Model file for the job. Use its own axes, mm. A direction names the side the tool comes from. Round coordinates to 2 decimals unless told otherwise and drop trailing zeros. Loops run counter-clockwise (first coordinate to the right, second up) from the corner with the lowest first, then second, coordinate; pieces in that order, holes last.
from build123d import *
from OCP.BRepFilletAPI import BRepFilletAPI_MakeChamfer

# Parameters (mm, degrees)
BOSS_EXTRUDE1_DEPTH = 11.1125
FILLET1_R           = 6.35
FILLET2_R           = 5.715
SKETCH2_R           = 2.794
BOSS_EXTRUDE2_DEPTH = 3.175
BOSS_EXTRUDE3_DEPTH = 1.27
SKETCH4_W           = 1.016
SKETCH4_H           = 4.445
CUT_EXTRUDE2_DEPTH  = 20.997176622
CHAMFER1_SIZE       = 0.79375
CHAMFER1_SIZE2      = 0.458271776


# Some blends are built 0.0001 mm under size
with BuildPart() as part:
    # Sketch1 → Boss-Extrude1 (new body)
    with BuildSketch(Plane.XY):
        with BuildLine():
            Line((3.302, 0), (15.367, 0))
            Line((15.367, 0), (15.367, -6.35))
            Line((15.367, -6.35), (-6.477, -6.35))
            Line((-6.477, -6.35), (-6.477, 0))
            Line((-6.477, 0), (-3.302, 0))
            ThreePointArc((-3.302, 0), (0, -3.302), (3.302, 0))
        make_face()
    extrude(amount=BOSS_EXTRUDE1_DEPTH)

    # Fillet1
    fillet1_edges = [part.edges().sort_by_distance(p)[0] for p in [
        (-6.477, -6.35, 5.55625),
    ]]
    fillet(fillet1_edges, radius=FILLET1_R - 0.0001)  # a hair under: the kernel refuses the full size

    # Fillet2
    # the kernel refuses this fillet: 5.715 mm, written as the material it takes off along each edge
    with BuildSketch(Plane(origin=(15.367, 14.2875, 0), x_dir=(-1, 0, 0), z_dir=(0, -1, 0)), Plane(origin=(15.367, 14.2875, 11.1125), x_dir=(0, 0, -1), z_dir=(0, -1, 0))) as fillet2_piece_1:
        with BuildLine():
            CenterArc((FILLET2_R, -FILLET2_R), FILLET2_R, 90, 90)
            Line((0, -FILLET2_R), (0, 0))
            Line((0, 0), (FILLET2_R, 0))
        make_face()
    extrude(amount=34.925, mode=Mode.SUBTRACT)

    # Sketch2 → Boss-Extrude2 (add)
    with BuildSketch(Plane(origin=(0, 0, 0), x_dir=(1, 0, 0), z_dir=(0, 1, 0))):
        with Locations(Location((9.652, -5.55625, 0), (0, 0, 270))):
            Circle(SKETCH2_R)
    extrude(amount=BOSS_EXTRUDE2_DEPTH)

    # Sketch3 → Boss-Extrude3 (add)
    with BuildSketch(Plane(origin=(0, 3.175, 0), x_dir=(1, 0, 0), z_dir=(0, 1, 0))):
        with BuildLine():
            Line((7.89223638, -8.35025), (11.41176362, -8.35025))
            ThreePointArc((11.41176362, -8.35025), (12.954, -5.55625), (11.41176362, -2.76225))
            Line((11.41176362, -2.76225), (7.89223638, -2.76225))
            ThreePointArc((7.89223638, -2.76225), (6.35, -5.55625), (7.89223638, -8.35025))
        make_face()
    extrude(amount=BOSS_EXTRUDE3_DEPTH)

    # Sketch4 → Cut-Extrude2 (cut, through all)
    with BuildSketch(Plane.XY):
        with Locations((9.652, 2.2225)):
            Rectangle(SKETCH4_W, SKETCH4_H)
    extrude(amount=CUT_EXTRUDE2_DEPTH, mode=Mode.SUBTRACT)

    # Chamfer1: one chamfer whose edges measure the first distance from different faces: ONE call of the kernel's chamfer builder (chamfer() names one face for all edges)
    chamfer1_edges_1 = [part.edges().sort_by_distance(p)[0] for p in [
        (6.35, 4.445, 5.55625),
    ]]
    chamfer1_side_1 = [part.faces().sort_by_distance(p)[0] for p in [
        (6.35, 3.81, 5.55625),
    ]]
    chamfer1_edges_2 = [part.edges().sort_by_distance(p)[0] for p in [
        (12.954, 4.445, 5.55625),
    ]]
    chamfer1_side_2 = [part.faces().sort_by_distance(p)[0] for p in [
        (12.954, 3.81, 5.55625),
    ]]
    chamfer1 = BRepFilletAPI_MakeChamfer(part.part.solid().wrapped)
    for e in chamfer1_edges_1:
        chamfer1.Add(CHAMFER1_SIZE, CHAMFER1_SIZE2, e.wrapped, chamfer1_side_1[0].wrapped)  # the first distance lies on this face
    for e in chamfer1_edges_2:
        chamfer1.Add(CHAMFER1_SIZE, CHAMFER1_SIZE2, e.wrapped, chamfer1_side_2[0].wrapped)  # the first distance lies on this face
    add(Compound.cast(chamfer1.Shape()), mode=Mode.REPLACE)


solid = part.part
Q1. Slice it at D-D on y = 0.5. Give the cut face in (x, z).
Q2. Tool access for faces 1 (the face through (9.144, 2, 6)), 2 (the face through (10.7, 3.7, 2.762)), 3 (the face through (-5, 0, 5)), 4 (the face through (6.86, 1.57, 5.5)): list every direction of +Z, -Z, +X, -X, +Y, -Y with a clear straight run to the whole face (end or side of a thin tool).
Q3. Slice it at C-C on x = 3.75. Give the cut face in (y, z).
Q4. Probe line 1 (Y direction, x = 6, z = 6.25); line 2 (X direction, y = -1, z = 7.75); line 3 (Z direction, x = 9.75, y = -2.75). List the from-to ranges inside material, lowest first.
Q5. Pull direction Y, two halves, no side cores. Call faces 5 (the face through (11, 4.445, 6)), 6 (the face through (13.592, -3.131, 1.575)), 7 (the face through (6.7, 3.175, 5.5)): pulls with the +Y half, pulls with the -Y half, needs draft (parallel to the pull), parting line crosses it, or undercut.
Q6. Flat gauge pins, fed straight in: P1, Ø1, axis at y = 3.5, z = 4, coming from the -X side; P2, Ø0.6, axis at x = 11, y = 3.5, coming from the -Z side; P3, Ø1.3, axis at y = 1.5, z = 5.5, coming from the -X side. Where does each tip first touch, or does it go through?
Q7. Slice it at A-A on y = -2.25. Give the cut face in (x, z) (1 decimal).
Reply:
1. outline: (9.14, 2.81) - (9.14, 8.3) arc R2.79 ccw to start; (10.16, 2.81) arc R2.79 ccw to (10.16, 8.3) - close
2. face 1: +Z, -Z, +Y
2. face 2: -Z, +X, -X, +Y
2. face 3: +Z, -Z, -X, +Y
2. face 4: -X
3. outline: (-6.35, 0) - (0, 0) - (0, 11.11) - (-6.35, 11.11) - close
4. line 1: y = -6.35 to 0
4. line 2: x = -6.4 to -3.15, 3.15 to 14.86
4. line 3: z = 0 to 11.11
5. face 5: pulls with the +Y half
5. face 6: needs draft
5. face 7: undercut
6. P1: stops at x = 6.52
6. P2: stops at z = 2.76
6. P3: stops at x = 6.86
7. outline: (-6.1, 0) - (-2.4, 0) - (-2.4, 11.1) - (-6.1, 11.1) - close; (2.4, 0) - (9.7, 0) arc R5.7 ccw to (15.4, 5.6) arc R5.7 ccw to (9.7, 11.1) - (2.4, 11.1) - close
